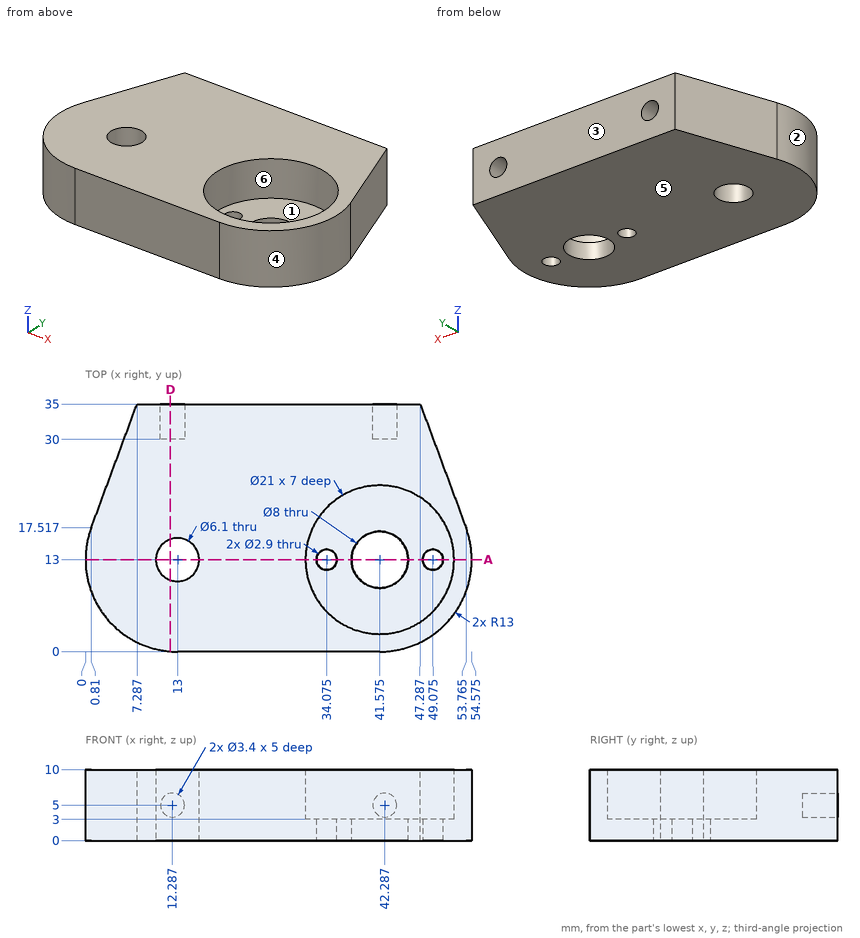
Could you check a few things on this drawing? It's one solid part, dimensions in mm from its lowest x, y, z. A direction names the side the tool comes from. Give positions to 0.01 mm unless a question says otherwise; leave off trailing zeros. Order: outer loops, then holes, each group sorted by start corner. A loop starts at its lowest first (then second) coordinate and runs counter-clockwise, first axis right, second up. Notation, with made-up numbers: (78.5, 69.25) - (125.5, 69.25) arc R36 cw to (125.5, 108.25) - close; hole circle Ø11 at (-1, 68). An arc over 180 degrees is marked (long way). Answer as a JSON object with one key per item and string values. Group by question number.
Item 1: For P1, Ø7, axis at x = 41.575, y = 13, coming from the +Z side; P2, Ø1.7, axis at x = 42, z = 5.5, coming from the +Y side, each with a flat end and sliding along its axis, tell me the tip position at first contact or that it passes through.
Item 2: Please list where these lines run through material, in increasing order: probe 1 along Y at (x, z) = (13, 7.5); probe 2 along X at (y, z) = (15, 1) (1 decimal); probe 3 along Y at (x, z) = (13, 5.75).
Item 3: If we mould it in two halves opening along X, with no side actions, what happens to the marked faces 1, 2, 3 and 4? For each: pulls with the +X half, pulls with the -X half, needs draft (parallel to the pull), parting line crosses it, or undercut.
Item 4: Which directions (+Z, -Z, +X, -X, +Y, -Y) give clear straight access to the entire face, cutting with the end or side of a thin tool? Please do the marked faces 5 and 6.
Item 5: If we section it at D-D on x = 12: Please give me the cut outline in (y, z) (1 decimal).
Item 6: If we section it at A-A on y = 13: Give the number of separate pieces and of enclosed holes in the cut face, and give its area (3 significant figures).
Result set:
{
 "1": {"P1": "through", "P2": "y = 30"},
 "2": {"probe 1": "0 to 9.95, 16.05 to 35", "probe 2": "0.2 to 10.7, 15.3 to 38.1, 45 to 54.4", "probe 3": "0 to 9.95, 16.05 to 30"},
 "3": {"face 1": "undercut", "face 2": "pulls with the -X half", "face 3": "needs draft", "face 4": "pulls with the +X half"},
 "4": {"face 5": "-Z, +X, -X, +Y, -Y", "face 6": "+Z"},
 "5": {"outline": "(0, 0) - (10.1, 0) - (10.1, 10) - (0, 10) - close; (15.9, 0) - (35, 0) - (35, 3.3) - (30, 3.3) - (30, 6.7) - (35, 6.7) - (35, 10) - (15.9, 10) - close"},
 "6": {"separate pieces": "5", "enclosed holes": "0", "area": "296 mm²"}
}
